Check sheet for the drawn part. Datum: minimum x, y, z corner. Units: mm. A direction names the side the tool comes from. Round coordinates to 2 decimals unless told otherwise and drop trailing zeros. Order: outer loops, then holes, each group sorted by start corner. A loop starts at its lowest first (then second) coordinate and runs counter-clockwise, first axis right, second up. Notation, with made-up numbers: (4, -8.75) -> (22, -8.75) arc R12 ccw to (22, 13.25) -> close; hole circle Ø3 at (39, 10). An arc over 180 degrees is marked (long way). Answer in a Markdown table with one row per item.
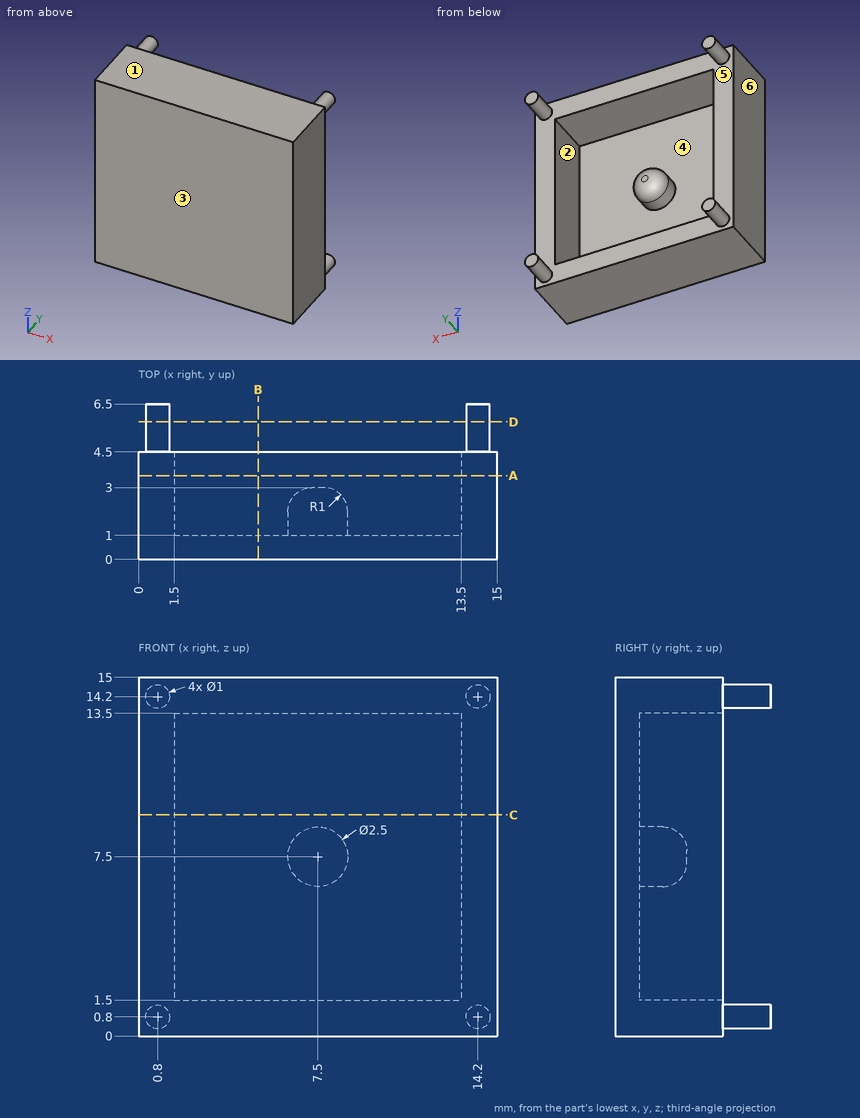
(1) Draft check along X on the marked faces 3, 4, 5 and 6. Enter one of: pulls with the +X half, pulls with the -X half, needs draft (parallel to the pull), parting line crosses it, or undercut.
Solutions:
| item | result |
|---|---|
| face 3 | needs draft |
| face 4 | undercut |
| face 5 | undercut |
| face 6 | pulls with the -X half |
(2) Section check A-A on y = 3.5. Record the boundary of the cut face in (x, z), plus the area to 3 significant figures.
Solutions:
| item | result |
|---|---|
| outline | (0, 0) -> (15, 0) -> (15, 15) -> (0, 15) -> close; hole (1.5, 1.5) -> (13.5, 1.5) -> (13.5, 13.5) -> (1.5, 13.5) -> close |
| area | 81.0 mm^2 |
(3) Tool access check on the marked faces 1 and 2. Record the directions out of +Z, -Z, +X, -X, +Y, -Y that give a thin tool (end or side, any length) a straight path to the whole face; none if there is none.
Solutions:
| item | result |
|---|---|
| face 1 | +Z, +X, -X, +Y, -Y |
| face 2 | +Y |
(4) Section check B-B on x = 5. Record the boundary of the cut face in (y, z).
Solutions:
| item | result |
|---|---|
| outline | (0, 0) -> (4.5, 0) -> (4.5, 1.5) -> (1, 1.5) -> (1, 13.5) -> (4.5, 13.5) -> (4.5, 15) -> (0, 15) -> close |
(5) Section check C-C on z = 9.25. Record the boundary of the cut face in (x, y), plus the area to 3 significant figures.
Solutions:
| item | result |
|---|---|
| outline | (0, 0) -> (15, 0) -> (15, 4.5) -> (13.5, 4.5) -> (13.5, 1) -> (1.5, 1) -> (1.5, 4.5) -> (0, 4.5) -> close |
| area | 25.5 mm^2 |
(6) Section check D-D on y = 5.75. Record the boundary of the cut face in (x, z).
Solutions:
| item | result |
|---|---|
| outline | circle Ø1 at (0.8, 0.8); circle Ø1 at (0.8, 14.2); circle Ø1 at (14.2, 0.8); circle Ø1 at (14.2, 14.2) |
(7) Scan lines: probe 1 along Z at (x, y) = (9, 3); probe 2 along Z at (x, y) = (7.5, 2.25). Record each from-to range of solid material in increasing order. Write a range as from..to.
Solutions:
| item | result |
|---|---|
| probe 1 | 0..1.5, 13.5..15 |
| probe 2 | 0..1.5, 6.28..8.72, 13.5..15 |
(8) Depth check by flat-ended pin: pin 1 Ø6 at (x, z) = (7.5, 8) entering from +Y. Enter the tip coordinate at first touch or a pass-through.
Solutions:
| item | result |
|---|---|
| pin 1 | y = 3 |
